```python
from build123d import *

# Parameters (mm, degrees)
BOSS_EXTRUDE1_DEPTH = 4
CUT_EXTRUDE1_DEPTH  = 2
FILLET1_R           = 0.5


with BuildPart() as part:
    # Sketch1 → Boss-Extrude1 (new body)
    with BuildSketch(Plane(origin=(0, 0, 0), x_dir=(1, 0, 0), z_dir=(0, 1, 0))):
        with BuildLine():
            ThreePointArc((-3.119170202, 8.456995758), (-9.456995758, 7.880829798), (-8.880829798, 1.543004242))
            ThreePointArc((-8.880829798, 1.543004242), (-7.531913687, 0.7687779), (-6, 0.5))
            Line((-6, 0.5), (-6, 3.4))
            ThreePointArc((-6, 3.4), (-7.13137085, 6.13137085), (-4.4, 5))
            Line((-4.4, 5), (-1.5, 5))
            ThreePointArc((-1.5, 5), (-1.924847604, 6.908699283), (-3.119170202, 8.456995758))
        make_face()
        with BuildLine():
            Line((-6, 3.4), (-6, 0.5))
            ThreePointArc((-6, 0.5), (-2.818019485, 1.818019485), (-1.5, 5))
            Line((-1.5, 5), (-4.4, 5))
            ThreePointArc((-4.4, 5), (-4.86862915, 3.86862915), (-6, 3.4))
        make_face()
        with BuildLine():
            Line((-6, 0.5), (-6, -0.857687257))
            Line((-6, -0.857687257), (-1.029224708, -5))
            Line((-1.029224708, -5), (1.5, -5))
            ThreePointArc((1.5, -5), (2.818019485, -1.818019485), (6, -0.5))
            Line((6, -0.5), (6, 0.857687257))
            Line((6, 0.857687257), (1.029224708, 5))
            Line((1.029224708, 5), (-1.5, 5))
            ThreePointArc((-1.5, 5), (-2.818019485, 1.818019485), (-6, 0.5))
        make_face()
        with BuildLine():
            ThreePointArc((1.5, -5), (1.924847604, -6.908699283), (3.119170202, -8.456995758))
            ThreePointArc((3.119170202, -8.456995758), (7.908699283, -9.075152396), (10.5, -5))
            ThreePointArc((10.5, -5), (10.075152396, -3.091300717), (8.880829798, -1.543004242))
            ThreePointArc((8.880829798, -1.543004242), (7.531913687, -0.7687779), (6, -0.5))
            Line((6, -0.5), (6, -3.4))
            ThreePointArc((6, -3.4), (7.13137085, -3.86862915), (7.6, -5))
            ThreePointArc((7.6, -5), (6, -6.6), (4.4, -5))
            Line((4.4, -5), (1.5, -5))
        make_face()
        with BuildLine():
            ThreePointArc((6, -0.5), (2.818019485, -1.818019485), (1.5, -5))
            Line((1.5, -5), (4.4, -5))
            ThreePointArc((4.4, -5), (4.86862915, -3.86862915), (6, -3.4))
            Line((6, -3.4), (6, -0.5))
        make_face()
        with BuildLine():
            Line((1.5, -5), (-1.029224708, -5))
            Line((-1.029224708, -5), (3.119170202, -8.456995758))
            ThreePointArc((3.119170202, -8.456995758), (1.924847604, -6.908699283), (1.5, -5))
        make_face()
        with BuildLine():
            ThreePointArc((-6, 0.5), (-7.531913687, 0.7687779), (-8.880829798, 1.543004242))
            Line((-8.880829798, 1.543004242), (-6, -0.857687257))
            Line((-6, -0.857687257), (-6, 0.5))
        make_face()
        with BuildLine():
            Line((8.880829798, -1.543004242), (6, 0.857687257))
            Line((6, 0.857687257), (6, -0.5))
            ThreePointArc((6, -0.5), (7.531913687, -0.7687779), (8.880829798, -1.543004242))
        make_face()
        with BuildLine():
            Line((1.029224708, 5), (-3.119170202, 8.456995758))
            ThreePointArc((-3.119170202, 8.456995758), (-1.924847604, 6.908699283), (-1.5, 5))
            Line((-1.5, 5), (1.029224708, 5))
        make_face()
    extrude(amount=BOSS_EXTRUDE1_DEPTH)

    # Sketch2 → Cut-Extrude1 (cut)
    with BuildSketch(Plane(origin=(0, 4, 0), x_dir=(1, 0, 0), z_dir=(0, 1, 0))):
        Polygon((-8.439430194, 7.032858495), (-8.980222196, 3.903820729), (-6.540792002, 1.870962234), (-3.560569806, 2.967141505), (-3.019777804, 6.096179271), (-5.459207998, 8.129037766), align=None)
        Polygon((5.459207998, -8.129037766), (3.019777804, -6.096179271), (3.560569806, -2.967141505), (6.540792002, -1.870962234), (8.980222196, -3.903820729), (8.439430194, -7.032858495), align=None)
    extrude(amount=-CUT_EXTRUDE1_DEPTH, mode=Mode.SUBTRACT)

    # Fillet1
    fillet1_edges = [part.edges().sort_by_distance(p)[0] for p in [
        (-2.880829798, 4, 3.456995758),
        (9.456995758, 4, 7.880829798),
        (2.880829798, 4, -3.456995758),
        (-9.456995758, 4, -7.880829798),
    ]]
    fillet(fillet1_edges, radius=FILLET1_R)


solid = part.part
```
For this review, take the finished solid that the model builds, in its own axes (mm). A direction names the side the tool comes from. Coordinates: 2 decimals unless noted, no trailing zeros. Write each loop counter-clockwise with the first axis right and the second up, starting at its lowest first coordinate (ties: lowest second). Pieces come first, ordered by that corner, then holes.
(1) The part is to be moulded in two halves that separate along Z. For faces 3 (the face through (0, 0, 0)), 4 (the face through (-3.294, 3.014, -4.51)), 5 (the face through (-7.778, 3.014, -2.902)), 6 (the face through (-9.39, 1.73, -7.96)), say which applies: +Z half, -Z half, draft (parallel to the pull), parting line (faces both ways), or undercut.
(2) Wall thickness on probe 1 along X at (y, z) = (1.7, 5); probe 2 along Z at (x, y) = (-6, 1.25); probe 3 along X at (y, z) = (1.3, -5): over which ranges is each line inside the solid? List them lowest first.
(3) Add section A-A on y = 0.45. Give the boundary of the cut face in (x, z).
(4) For pin 1 Ø3.5 at (x, z) = (-6, -5) entering from -Y; pin 2 Ø1.8 at (x, z) = (-5, -4) entering from +Y; pin 3 Ø1 at (y, z) = (2, -6.5) entering from +X, all flat-tipped, find the tip position at first contact; note any pin that passes through.
(5) Tool access review of faces 1 (the face through (8.714, 3.014, 5.446)), 2 (the face through (0, 4, 1)): name each direction out of +Z, -Z, +X, -X, +Y, -Y from which nothing blocks a thin tool from reaching the whole face with its end or side.
Answer sheet:
1. face 3: draft
1. face 4: undercut
1. face 5: undercut
1. face 6: parting line
2. probe 1: x = -1.03 to 4.4, 7.6 to 10.5
2. probe 2: z = -9.5 to -6.6, -3.4 to 0.86
2. probe 3: x = -10.5 to -7.6, -4.4 to 1.03
3. outline: (-8.88, -1.54) arc R4.5 ccw to (-3.12, -8.46) - (8.88, 1.54) arc R4.5 ccw to (3.12, 8.46) - close; hole circle Ø3.2 at (-6, -5); hole circle Ø3.2 at (6, 5)
4. pin 1: stops at y = 0
4. pin 2: stops at y = 2
4. pin 3: stops at x = -0.17
5. face 1: +Y
5. face 2: +Z, -Z, +X, -X, +Y
